Autodesk Inventor part; units mm, degrees
ref_plane "YZ Plane" through (0, 0, 0) normal (1, 0, 0) x (0, 1, 0)
ref_plane "XZ Plane" through (0, 0, 0) normal (0, 1, 0) x (-1, 0, 0)
ref_plane "XY Plane" through (0, 0, 0) normal (0, 0, 1) x (1, 0, 0)
sketch "Sketch1" plane through (0, 0, 0) normal (0, 0, 1) x (1, 0, 0)
  line L0 (0, 0) -> (70, 0)
  line L1 (70, 0) -> (70, -12)
  line L2 (70, -12) -> (0, -12)
  line L3 (0, -12) -> (0, 0)
  line L4 (70, 0) -> (50, 0)
  line L5 (50, 0) -> (50, 7.5)
  line L6 (50, 7.5) -> (70, 7.5)
  line L7 (70, 7.5) -> (70, 0)
  circle A0 centre (60, -2.25) radius 2.5
  point P0 (0, -6)
  point P1 (70, -6)
  point P2 (35, 0)
  point P3 (50, 0)
  dimension "d0" = 70
  dimension "d1" = 12
  dimension "d11" = 20
  dimension "d12" = 7.5
  dimension "d15" = 9.75
  dimension "d16" = 10
  dimension "d17" = 5
extrude "Extrusion2" add sketch "Sketch1" along normal blind 5 contours L0 A0 L1 L2 L3 | L5 L6 L7 L0 A0
properties part number "Touchscreen mount v03"
The listing builds one solid part. Answer for the finished solid, in the listing's coordinates (mm). A direction names the side the tool comes from. Round coordinates to 2 decimals unless told otherwise and drop trailing zeros. Write each loop counter-clockwise with the first axis right and the second up, starting at its lowest first coordinate (ties: lowest second). Pieces come first, ordered by that corner, then holes. Notation, with made-up numbers: M 24,15 L 49,15 A27 ccw 49,51 Z; hole C 80.25,79.5 d9. An arc over 180 degrees is marked long. Write each question's results on one line, items separated by ' | '. Start each with the question number.
(1) For faces 1 (the flat face through (42, -4, 0)), 2 (the flat face through (50, 4, 2)), determine the directions among +Z, -Z, +X, -X, +Y, -Y from which every point of the face is accessible in a straight line to the end or side of a thin tool.
(2) The part is cut by section B-B, the plane y = -2.25. Write down the section's boundary in (x, z), and give its area (3 significant figures).
(3) The part is cut by section D-D, the plane y = 4.25. Write down the section's boundary in (x, z), and give its area (3 significant figures).
(4) The part is cut by section C-C, the plane z = 2.3. Write down the section's boundary in (x, y).
(5) Each of these flat-tipped pins is pushed along its axis until it touches: P1, Ø2.5, axis at y = 4, z = 3.5, coming from the -X side; P2, Ø2.5, axis at x = 34.5, z = 1.5, coming from the +Y side. Where does it stop, or does it pass through?
(6) Determine the mould class of faces 3 (the cylindrical face through (62.31, -1.29, 2.46)), 4 (the flat face through (42, -4, 5)), 5 (the flat face through (35, -12, 2)) for opening direction Y: +Y half, -Y half, draft (parallel to the pull), parting line (faces both ways), or undercut.
(7) The part is cut by section A-A, the plane x = 60. Write down the section's boundary in (y, z), and give its area (3 significant figures).
(8) Find the intervals of material crossed by line 1 (X direction, y = -2.25, z = 2.65); line 2 (Y direction, x = 60, z = 1.4); line 3 (Y direction, x = 47, z = 2.15), in increasing order.
Worked answers:
1) face 1: -Z, +X, -X, +Y, -Y | face 2: +Z, -Z, -X, +Y
2) outline: M 0,0 L 57.5,0 L 57.5,5 L 0,5 Z; M 62.5,0 L 70,0 L 70,5 L 62.5,5 Z | area: 325 mm²
3) outline: M 50,0 L 70,0 L 70,5 L 50,5 Z | area: 100 mm²
4) outline: M 0,-12 L 70,-12 L 70,7.5 L 50,7.5 L 50,0 L 0,0 Z; hole C 60,-2.25 d5
5) P1: stops at x = 50 | P2: stops at y = 0
6) face 3: undercut | face 4: draft | face 5: -Y half
7) outline: M -12,0 L -4.75,0 L -4.75,5 L -12,5 Z; M 0.25,0 L 7.5,0 L 7.5,5 L 0.25,5 Z | area: 72.5 mm²
8) line 1: x = 0 to 57.5, 62.5 to 70 | line 2: y = -12 to -4.75, 0.25 to 7.5 | line 3: y = -12 to 0
